Part print with two shaded views. Sizes in mm from the minimum x, y, z corner. A direction names the side the tool comes from. Round coordinates to 2 decimals unless told otherwise and drop trailing zeros. Order: outer loops, then holes, each group sorted by start corner. A loop starts at its lowest first (then second) coordinate and runs counter-clockwise, first axis right, second up. Notation, with made-up numbers: (-25, 59.25) -> (-15, 59.25) arc R16 ccw to (-15, 74.25) -> close; hole circle Ø4 at (71.5, -2.75). An arc over 180 degrees is marked (long way). Answer as a JSON object with one key per item and string values.
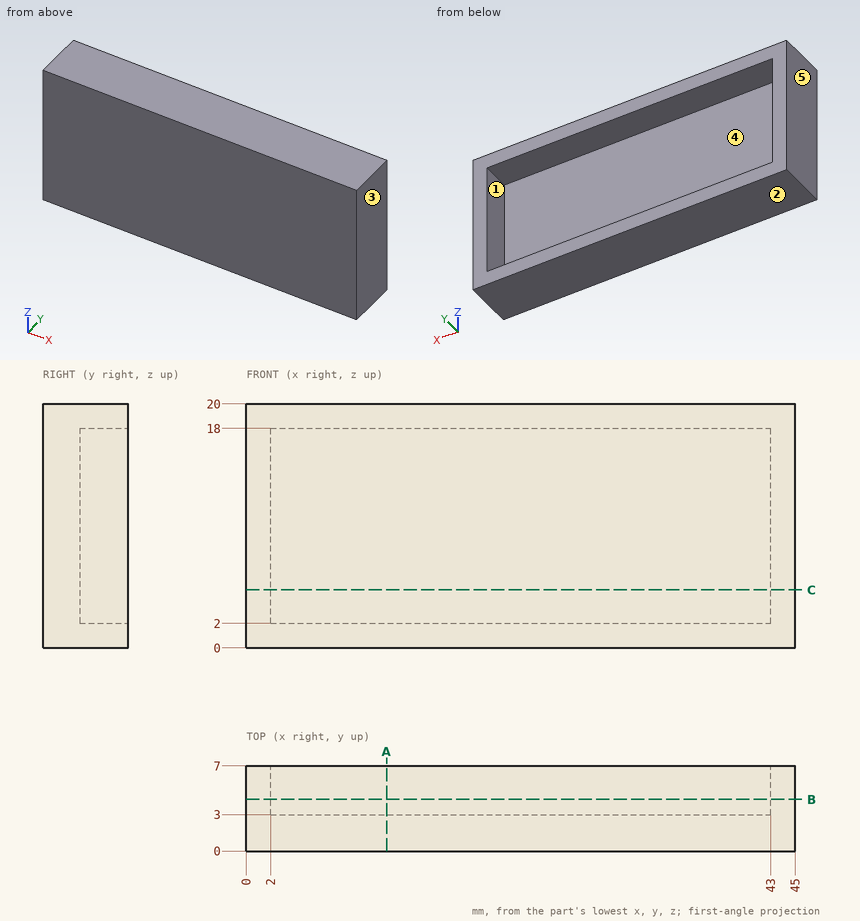
1) Cut at C-C, the plane z = 4.75. Give the cut face in (x, y).
Checked values:
{"outline": "(0, 0) -> (45, 0) -> (45, 7) -> (43, 7) -> (43, 3) -> (2, 3) -> (2, 7) -> (0, 7) -> close"}
2) Probe L1, parallel to Z at x = 27, y = 3.75; L2, parallel to X at y = 5.75, z = 14; L3, parallel to Y at x = 30, z = 7.75. List the from-to ranges inside material, lowest first. Write a range as from..to.
Checked values:
{"L1": "z = 0..2, 18..20", "L2": "x = 0..2, 43..45", "L3": "y = 0..3"}
3) Which spindle directions (+Z, -Z, +X, -X, +Y, -Y) get a long thin tool onto all of the face, cutting with end or side? Do the marked faces 4 and 5. Say none if no direction does.
Checked values:
{"face 4": "+Y", "face 5": "+Z, -Z, -X, +Y, -Y"}
4) Cut at A-A, the plane x = 11.5. Give the cut face in (y, z), plus the area to 3 significant figures.
Checked values:
{"outline": "(0, 0) -> (7, 0) -> (7, 2) -> (3, 2) -> (3, 18) -> (7, 18) -> (7, 20) -> (0, 20) -> close", "area": "76.0 mm²"}
5) Cut at B-B, the plane y = 4.25. Give the cut face in (x, z), plus the area to 3 significant figures.
Checked values:
{"outline": "(0, 0) -> (45, 0) -> (45, 20) -> (0, 20) -> close; hole (2, 2) -> (43, 2) -> (43, 18) -> (2, 18) -> close", "area": "244 mm²"}
6) Pull direction X, two halves, no side cores. Call the marked faces 1, 2 and 3: pulls with the +X half, pulls with the -X half, needs draft (parallel to the pull), parting line crosses it, or undercut.
Checked values:
{"face 1": "undercut", "face 2": "needs draft", "face 3": "pulls with the +X half"}
